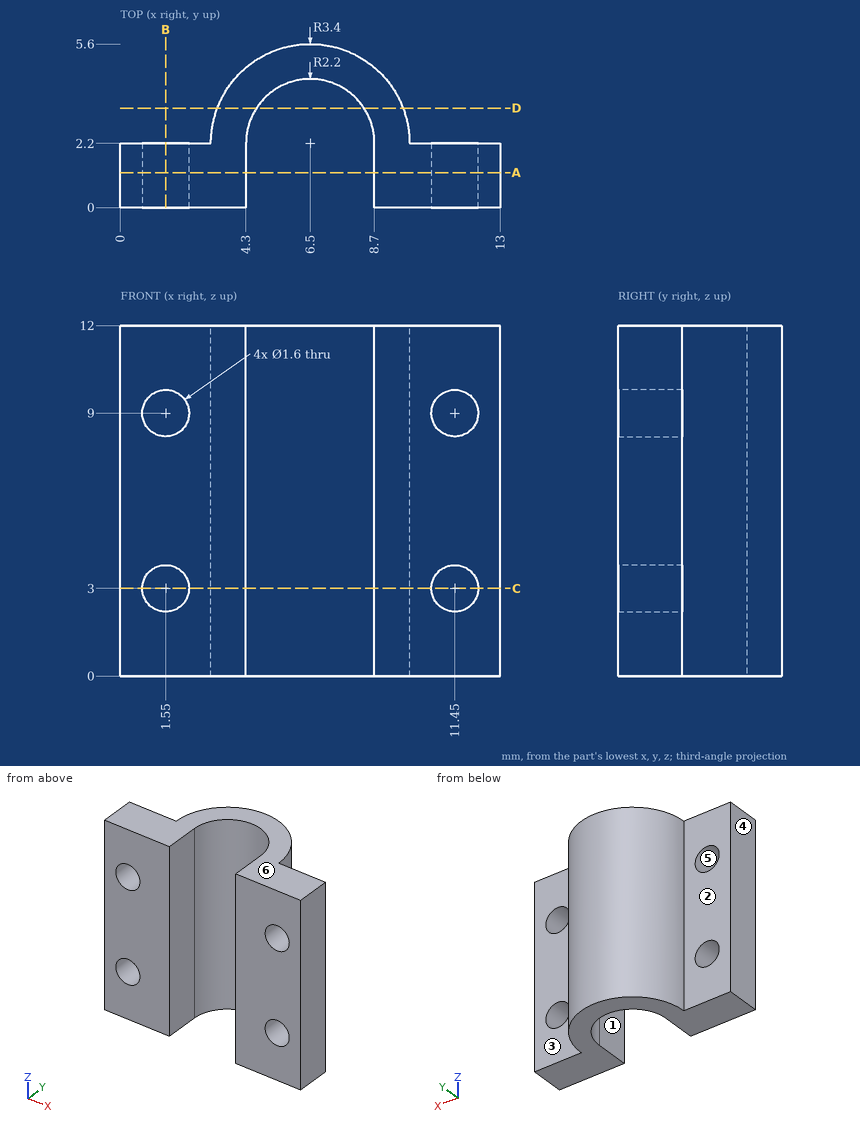
Geometry check sheet. Reference: drawing and pictorial views, mm from the part's lowest x, y, z. A direction names the side the tool comes from. Give positions to 0.01 mm unless a question says otherwise; leave off trailing zeros. Write each loop counter-clockwise with the first axis right and the second up, starting at its lowest first coordinate (ties: lowest second). Pieces come first, ordered by that corner, then holes.
Item 1: Scan lines: L1, parallel to X at y = 1.7, z = 8.75; L2, parallel to X at y = 0.5, z = 2.5; L3, parallel to X at y = 2.15, z = 6. Record each from-to range of solid material in increasing order.
Item 2: Draft check along X on the marked faces 4, 5 and 6. Enter one of: released by +X, released by -X, zero draft, split by the parting line, or undercut.
Item 3: Cross-section at A-A (y = 1.2). Enter the section's corners in (x, z), and give its area (3 significant figures).
Item 4: Gauge pin test, flat ends, axial feed: pin 1 (2.5 mm diameter, centred on x = 1.55, z = 9, fed in from +Y); pin 2 (3.5 mm diameter, centred on x = 2, z = 7, fed in from +Y); pin 3 (1.5 mm diameter, centred on x = 6.5, z = 4.5, fed in from -Y). Record the tip position at first contact, or that the pin passes through.
Item 5: Access from +Z, -Z, +X, -X, +Y, -Y to the whole of each face (thin tool, end or side, straight path). Record for the marked faces 1, 2 and 3.
Item 6: Cross-section at D-D (y = 3.4). Enter the section's corners in (x, z), and give its area (3 significant figures).
Item 7: Cross-section at B-B (x = 1.55). Enter the section's corners in (y, z).
Item 8: Cross-section at C-C (z = 3). Enter the section's corners in (x, y).
Report:
1. L1: x = 0 to 0.79, 2.31 to 4.3, 8.7 to 10.69, 12.21 to 13
1. L2: x = 0 to 0.93, 2.17 to 4.3, 8.7 to 10.83, 12.07 to 13
1. L3: x = 0 to 4.3, 8.7 to 13
2. face 4: released by -X
2. face 5: undercut
2. face 6: zero draft
3. outline: (0, 0) - (4.3, 0) - (4.3, 12) - (0, 12) - close; (8.7, 0) - (13, 0) - (13, 12) - (8.7, 12) - close; hole circle Ø1.6 at (1.55, 3); hole circle Ø1.6 at (1.55, 9); hole circle Ø1.6 at (11.45, 3); hole circle Ø1.6 at (11.45, 9)
3. area: 95.2 mm2
4. pin 1: stops at y = 2.2
4. pin 2: stops at y = 4.2
4. pin 3: stops at y = 4.27
5. face 1: +Z, -Z, -Y
5. face 2: +Z, -Z, -X, +Y
5. face 3: +Z, -Z, +X, +Y
6. outline: (3.32, 0) - (4.66, 0) - (4.66, 12) - (3.32, 12) - close; (8.34, 0) - (9.68, 0) - (9.68, 12) - (8.34, 12) - close
6. area: 32.1 mm2
7. outline: (0, 0) - (2.2, 0) - (2.2, 2.2) - (0, 2.2) - close; (0, 3.8) - (2.2, 3.8) - (2.2, 8.2) - (0, 8.2) - close; (0, 9.8) - (2.2, 9.8) - (2.2, 12) - (0, 12) - close
8. outline: (0, 0) - (0.75, 0) - (0.75, 2.2) - (0, 2.2) - close; (2.35, 0) - (4.3, 0) - (4.3, 2.2) arc R2.2 cw to (8.7, 2.2) - (8.7, 0) - (10.65, 0) - (10.65, 2.2) - (9.9, 2.2) arc R3.4 ccw to (3.1, 2.2) - (2.35, 2.2) - close; (12.25, 0) - (13, 0) - (13, 2.2) - (12.25, 2.2) - close
